Here's how the part is built. I have some questions about the finished solid (model axes, mm). Round coordinates to 2 decimals unless told otherwise and drop trailing zeros. Loops run counter-clockwise (first coordinate to the right, second up) from the corner with the lowest first, then second, coordinate; pieces in that order, holes last. Notation, with made-up numbers: M 44,-6.5 L 75,-6.5 A21 ccw 75,16.5 Z; hole C 45,58 d10. An arc over 180 degrees is marked long. Use a Markdown table: item, result.
Autodesk Fusion 360 part; units mm, degrees
sketch "Sketch1" plane through (0, 0, 0) normal (0, 0, 1) x (1, 0, 0)
  circle A0 centre (0, 0) radius 4
  dimension "d1" = 8
extrude "Extrude1" add sketch "Sketch1" along normal blind 8
sketch "Sketch2" plane through (0, 0, 8) normal (0, 0, 1) x (-1, 0, 0)
  circle A0 centre (0, 0) radius 4
  circle A1 centre (0, 0) radius 2.375
  dimension "d4" = 4.75
extrude "Extrude2" cut sketch "Sketch2" against normal blind 3 contours A1
sketch "Sketch3" plane through (0, 0, 5) normal (0, 0, 1) x (-1, 0, 0)
  circle A0 centre (0, 0) radius 2.375
  circle A1 centre (0, 0) radius 1.5
  dimension "d7" = 3
extrude "Extrude3" cut sketch "Sketch3" against normal blind 9 contours A1
sketch "Sketch4" plane through (0, 0, 8) normal (0, 0, 1) x (-1, 0, 0)
  circle A0 centre (0, 0) radius 2.375
  circle A1 centre (0, 0) radius 4
  circle A2 centre (0, 0) radius 6.5
  dimension "d10" = 13
extrude "Extrude4" add sketch "Sketch4" against normal blind 2 contours A2
extrude "Extrude5" add 1 faces at (3.1462, -0.2732, 0) along direction (0, 0, -1) blind 2
sketch "Sketch5" plane through (0, 0, -2) normal (0, 0, -1) x (1, 0, 0)
  circle A0 centre (0, 0) radius 1.5
  circle A1 centre (0, 0) radius 4
  circle A2 centre (0, 0) radius 3.2
  dimension "d18" = 6.4
extrude "Extrude6" cut sketch "Sketch5" against normal blind 0.5 contours A1
extrude "Extrude7" add 1 faces at (2.6214, 0.159, -2) along direction (0, 0, -1) blind 0.5
extrude "Extrude8" add 1 faces at (3.7184, 0.1987, -1.5) along direction (0, 0, -1) blind 0.5
extrude "Extrude9" cut 1 faces at (-2.0745, 0.118, 5) along direction (0, 0, -1) blind 3
extrude "Extrude10" cut 1 faces at (-2.0745, 0.118, 2) along direction (0, 0, -1) blind 1.5
extrude "Extrude11" add 1 faces at (3.7184, 0.1987, -2) along direction (0, 0, -1) blind 0.5
chamfer "Chamfer3" distance 0.43 angle 45 2 edges at (1.3985, 0.5424, 0.5) (2.2143, -0.8588, 0.5)
extrude "Extrude12" cut 1 faces at (3.1462, 0.2732, -2.5) along direction (0, 0, 1) blind 1.5
extrude "Extrude13" cut 1 faces at (-5.092, 0.4409, 8) along direction (0, 0, -1) blind 0.5
fillet "Fillet2" radius 0.5 2 edges at (2.2143, 0.8588, 7.5) (6.0601, -2.3505, 7.5)
Q1. Will this pin go through, and if not, where does the flat tip stop? P1, Ø5, axis at x = 0, y = 0, coming from the -Z side.
Return value:
| item | result |
|---|---|
| P1 | stops at z = -1 |
Q2. Imagine slicing it at A-A, the plane x = 0. Please give me the cut outline in (y, z) (3 decimals), then the cut area to 3 significant figures.
Return value:
| item | result |
|---|---|
| outline | M -6.5,6 L -4,6 L -4,-1 L -1.5,-1 L -1.5,0.07 L -1.93,0.5 L -1.945,0.5 L -2.375,0.93 L -2.375,7 A0.5 ccw -2.875,7.5 L -6,7.5 A0.5 ccw -6.5,7 Z; M 1.5,-1 L 4,-1 L 4,6 L 6.5,6 L 6.5,7 A0.5 ccw 6,7.5 L 2.875,7.5 A0.5 ccw 2.375,7 L 2.375,0.93 L 1.945,0.5 L 1.93,0.5 L 1.5,0.07 Z |
| area | 37.5 mm^2 |
Q3. I need wall thicknesses on line 1 (X direction, y = 0, z = -0.25); line 2 (Y direction, x = 0, z = 4) (3 decimals). Which ranges of each line are inside material? Lowest first, please. Write a range as from..to.
Return value:
| item | result |
|---|---|
| line 1 | x = -4..-1.5, 1.5..4 |
| line 2 | y = -4..-2.375, 2.375..4 |
Q4. We'd pull the mould along X, two halves only. Please class faces 1 (the flat face through (-3, -3, 6)), 2 (the cylindrical face through (-1.096, 2.107, 4.007)), 3 (the cylindrical face through (-0.867, -3.905, 2.549)): pulls with the +X half, pulls with the -X half, needs draft (parallel to the pull), parting line crosses it, or undercut.
Return value:
| item | result |
|---|---|
| face 1 | needs draft |
| face 2 | undercut |
| face 3 | parting line crosses it |
Q5. Imagine slicing it at C-C, the plane z = 4.5. Please give me the cut outline in (x, y) (3 decimals), then the cut area to 3 significant figures.
Return value:
| item | result |
|---|---|
| outline | C 0,0 d8; hole C 0,0 d4.75 |
| area | 32.5 mm^2 |
